Here's the drawing with two shaded views (mm, measured from the low corner). I have some questions. Round coordinates to 2 decimals unless told otherwise and drop trailing zeros. Write each loop counter-clockwise with the first axis right and the second up, starting at its lowest first coordinate (ties: lowest second). Pieces come first, ordered by that corner, then holes. Notation, with made-up numbers: M -16,-20 L 27,-20 A17 ccw 27,-15 Z; hole C 53,23.25 d9. An arc over 180 degrees is marked long. Write item = value, one per line. Start each with the question number.
(1) I need wall thicknesses on line 1 along Z through (x, y) = (47, 2.8); line 2 along X through (y, z) = (2.45, 17); line 3 along Z through (x, y) = (20.5, 1.95). Which ranges of each line are inside material? Lowest first, please.
(2) I want a section at A-A (y = 1.75). List the corners of the cut face in (x, z) for me, and give its area (3 significant figures).
(3) I want a section at B-B (x = 47). List the corners of the cut face in (y, z) for me, and give its area (3 significant figures).
(4) Will these pins go through, and if not, where does the flat tip stop? pin 1 Ø12 at (x, z) = (28, 11.5) entering from -Y; pin 2 Ø1.5 at (x, y) = (16, 4.5) entering from -Z; pin 3 Ø2 at (y, z) = (0.5, 71) entering from +X.
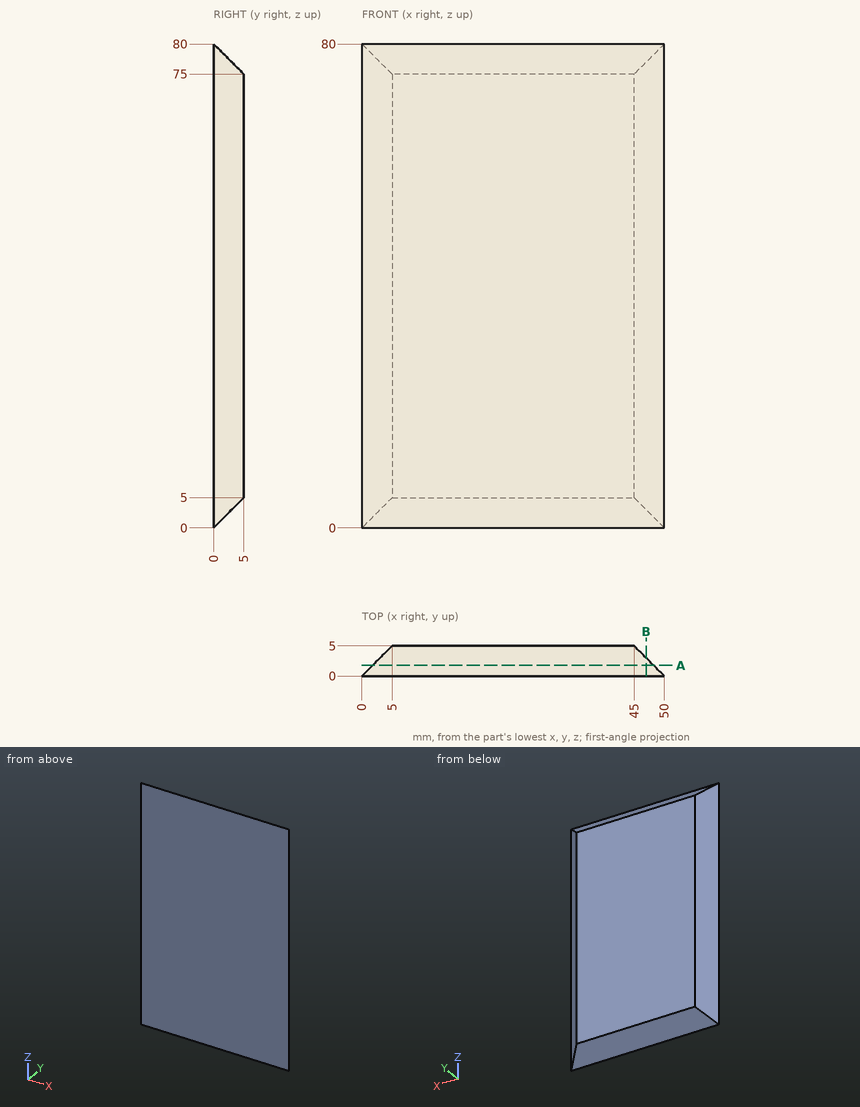
Returned:
q1.line_1 = 2.8 to 77.2
q1.line_2 = 2.45 to 47.55
q1.line_3 = 1.95 to 78.05
q2.outline = M 1.75,1.75 L 48.25,1.75 L 48.25,78.25 L 1.75,78.25 Z
q2.area = 3,560 mm²
q3.outline = M 0,0 L 3,3 L 3,77 L 0,80 Z
q3.area = 231 mm²
q4.pin_1 = 0
q4.pin_2 = 3.75
q4.pin_3 = 50
